Verification items for the finished model (mm, model axes). Face numbers are marked on the shaded views. A direction names the side the tool comes from. Give positions to 0.01 mm unless a question says otherwise; leave off trailing zeros. Write each loop counter-clockwise with the first axis right and the second up, starting at its lowest first coordinate (ties: lowest second). Pieces come first, ordered by that corner, then holes. Notation, with made-up numbers: (64.25, -3.5) - (121.25, -3.5) arc R23 ccw to (121.25, 34.5) - close; hole circle Ø4 at (32.5, 44). An arc over 180 degrees is marked (long way). Answer as a JSON object with one key per item and string values. Group by question number.
Item 1: Scan lines: line 1 along X through (y, z) = (1.75, -3); line 2 along X through (y, z) = (-3.5, -2); line 3 along Y through (x, z) = (-3.25, 5). Record each from-to range of solid material in increasing order. Write a range as [from, to].
Item 2: Go/stop test with flat-tipped pins: pin 1 (3.5 mm diameter, centred on y = 1, z = -4, fed in from +X); pin 2 (2.5 mm diameter, centred on y = 4, z = -3, fed in from -X); pin 3 (1.7 mm diameter, centred on x = 3.5, y = 8.5, fed in from +Z). Record where each tip stops, or that it passes through.
Item 3: Sectioned sample at D-D, the plane x = 4. Record the boundary of the cut face in (y, z), and give its area (3 significant figures).
Item 4: Tool access check on the marked faces 5, 6, 7 and 8. Record the directions out of +Z, -Z, +X, -X, +Y, -Y that give a thin tool (end or side, any length) a straight path to the whole face; none if there is none.
Item 5: Sectioned sample at B-B, the plane y = 1.5. Record the boundary of the cut face in (x, z), and give its area (3 significant figures).
Item 6: Draft check along X on the marked faces 1, 2, 3 and 4. Enter one of: +X half, -X half, draft (parallel to the pull), parting line (faces both ways), or undercut.
Item 7: Sectioned sample at A-A, the plane z = -3.75. Record the boundary of the cut face in (x, y).
```python
from build123d import *

# Parameters (mm, degrees)
F1_DEPTH = 7
F2_DEPTH = 6
F3_DEPTH = 15


with BuildPart() as f1:
    # F0 (on Front) → F1 (new body)
    with BuildSketch(Plane.XZ):
        with BuildLine():
            ThreePointArc((-3.477884, 0.719832), (-3.596369, -0.44229), (-3.343322, -1.5827))
            Line((-3.343322, -1.5827), (-3.322458, -1.593981))
            Line((-3.322458, -1.593981), (-3.322458, -2.283465))
            Line((-3.322458, -2.283465), (-2.589551, -2.283465))
            Line((-2.589551, -2.283465), (-2.176465, -2.283465))
            Line((-2.176465, -2.283465), (-2.176465, -1.823074))
            ThreePointArc((-2.176465, -1.823074), (0.063946, 2.521621), (2.304358, -1.823074))
            Line((2.304358, -1.823074), (2.304358, -2.283465))
            Line((2.304358, -2.283465), (2.717444, -2.283465))
            Line((2.717444, -2.283465), (3.450351, -2.283465))
            Line((3.450351, -2.283465), (3.450351, -1.634055))
            ThreePointArc((3.450351, -1.634055), (3.72254, -0.469953), (3.605777, 0.719832))
            ThreePointArc((3.605777, 0.719832), (2.307299, 2.6718), (0.091662, 3.438077))
            ThreePointArc((0.091662, 3.438077), (-2.157419, 2.688675), (-3.477884, 0.719832))
        make_face()
        Polygon((-3.322458, -2.283465), (-3.322458, -1.593981), (-4.089551, -1.943924), (-4.089551, -2.283465), align=None)
        with BuildLine():
            Line((-5.413338, 3.472093), (-3.477884, 0.719832))
            ThreePointArc((-3.477884, 0.719832), (-2.157419, 2.688675), (0.091662, 3.438077))
            Line((0.091662, 3.438077), (-4.408209, 3.472093))
            Line((-4.408209, 3.472093), (-1.413338, 5.938077))
            Line((-1.413338, 5.938077), (-5.413338, 5.938077))
            Line((-5.413338, 5.938077), (-5.413338, 3.472093))
        make_face()
        Polygon((-2.589551, -2.283465), (-3.322458, -2.283465), (-4.089551, -2.283465), (-4.089551, -4.949721), (-3.322458, -4.949721), (-2.589551, -4.949721), align=None)
        with BuildLine():
            Line((4.591534, 3.404061), (0.091662, 3.438077))
            ThreePointArc((0.091662, 3.438077), (2.307299, 2.6718), (3.605777, 0.719832))
            Line((3.605777, 0.719832), (5.587751, 3.472093))
            Line((5.587751, 3.472093), (5.587751, 5.938077))
            Line((5.587751, 5.938077), (1.596662, 5.938077))
            Line((1.596662, 5.938077), (4.591534, 3.404061))
        make_face()
        Polygon((-4.408209, 3.472093), (0.091662, 3.438077), (4.591534, 3.404061), (1.596662, 5.938077), (-1.413338, 5.938077), align=None)
        Polygon((4.217444, -1.943924), (3.450351, -1.634055), (3.450351, -2.283465), (4.217444, -2.283465), align=None)
        Polygon((4.217444, -2.283465), (3.450351, -2.283465), (2.717444, -2.283465), (2.717444, -4.949721), (3.450351, -4.949721), (4.217444, -4.949721), align=None)
    extrude(amount=F1_DEPTH)

    # F0 (on Front) → F2 (cut)
    with BuildSketch(Plane.XZ):
        Polygon((-4.408209, 3.472093), (0.091662, 3.438077), (4.591534, 3.404061), (1.596662, 5.938077), (-1.413338, 5.938077), align=None)
    extrude(amount=F2_DEPTH, mode=Mode.SUBTRACT)

    # F0 (on Front) → F3 (join)
    with BuildSketch(Plane.XZ):
        Polygon((4.217444, -2.283465), (3.450351, -2.283465), (2.717444, -2.283465), (2.717444, -4.949721), (3.450351, -4.949721), (4.217444, -4.949721), align=None)
        Polygon((-2.589551, -2.283465), (-3.322458, -2.283465), (-4.089551, -2.283465), (-4.089551, -4.949721), (-3.322458, -4.949721), (-2.589551, -4.949721), align=None)
    extrude(amount=-F3_DEPTH)


solid = f1.part
```
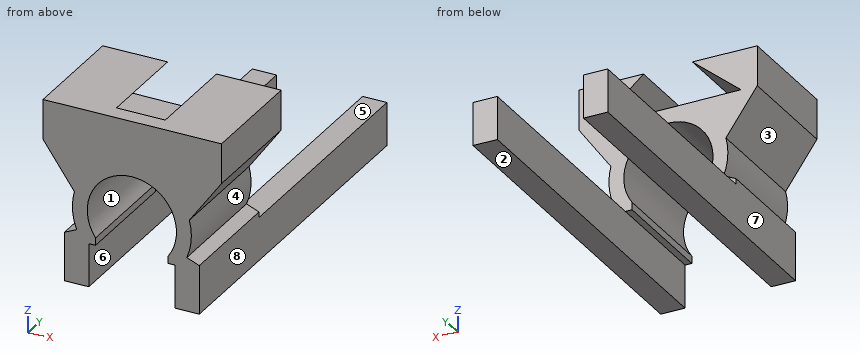
Geometry check:
{
 "1": {"line 1": "[-4.09, -2.59], [2.72, 4.22]", "line 2": "[-4.09, -2.18], [2.3, 4.22]", "line 3": "[-7, 0]"},
 "2": {"pin 1": "x = 4.22", "pin 2": "x = -4.09", "pin 3": "z = -2.28"},
 "3": {"outline": "(-7, -4.95) - (15, -4.95) - (15, -2.28) - (0, -2.28) - (0, -1.86) - (-7, -1.86) - close; (-7, 1.27) - (0, 1.27) - (0, 3.41) - (-6, 3.41) - (-6, 3.9) - (0, 3.9) - (0, 5.94) - (-7, 5.94) - close", "area": "91.4 mm^2"},
 "4": {"face 5": "+Z, +X, -X, +Y", "face 6": "-Z, +Y, -Y", "face 7": "-Z, -X, +Y, -Y", "face 8": "-Z, +X, +Y, -Y"},
 "5": {"outline": "(-4.09, -4.95) - (-2.59, -4.95) - (-2.59, -2.28) - (-4.09, -2.28) - close; (2.72, -4.95) - (4.22, -4.95) - (4.22, -2.28) - (2.72, -2.28) - close", "area": "8.00 mm^2"},
 "6": {"face 1": "undercut", "face 2": "draft", "face 3": "-X half", "face 4": "+X half"},
 "7": {"outline": "(-4.09, -7) - (-2.59, -7) - (-2.59, 15) - (-4.09, 15) - close; (2.72, -7) - (4.22, -7) - (4.22, 15) - (2.72, 15) - close"}
}
